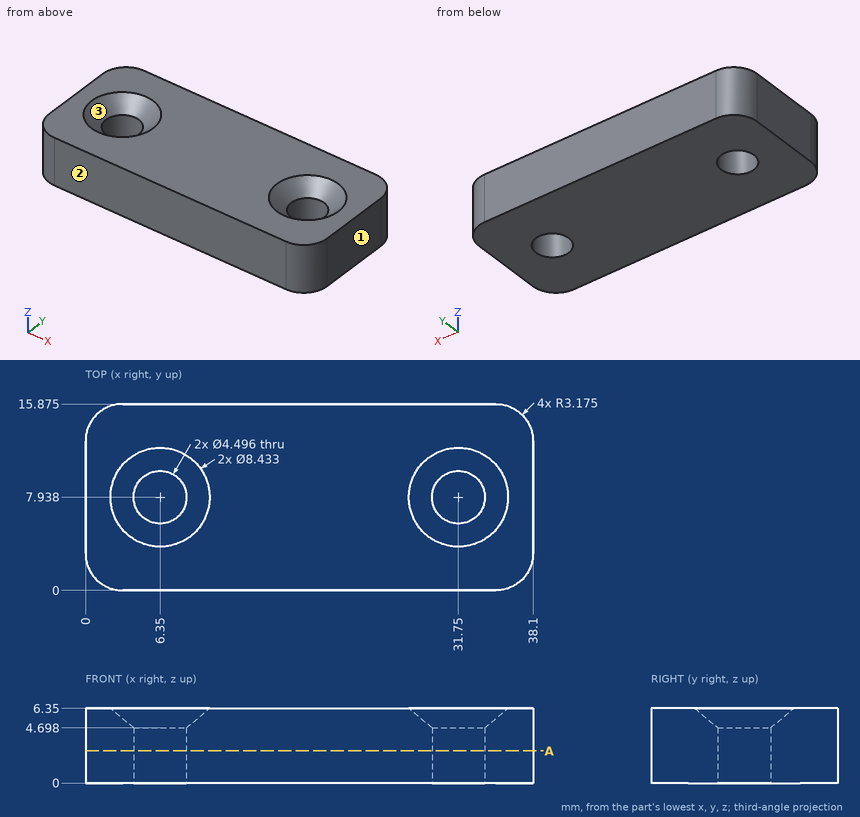
Design review of the part shown in the three views and the two pictorial views. Dimensions are in mm from the part's minimum x, y and z. Round coordinates to 2 decimals unless told otherwise and drop trailing zeros. Use one line per item in the form item = value.
1) Mouldability with a two-part tool opening along Y and no side actions: class the marked faces 1, 2 and 3 as pulls with the +Y half, pulls with the -Y half, needs draft (parallel to the pull), parting line crosses it, or undercut.
Solutions:
face_1 = needs draft
face_2 = pulls with the -Y half
face_3 = undercut
2) Clearance check with a flat-ended pin moving along its axis: P1, Ø1.5, axis at x = 13, z = 1, coming from the -Y side. State where the tip first meets the part, or that it passes through.
Solutions:
P1 = 0
3) We need section A-A on z = 2.75. State how many separate pieces and enclosed holes the cut face has.
Solutions:
separate_pieces = 1
enclosed_holes = 2
4) Wall thickness on probe 1 along Y at (x, z) = (31.75, 2.5) (1 decimal); probe 2 along X at (y, z) = (9, 3.5); probe 3 along X at (y, z) = (3, 3) (1 decimal): over which ranges is each line inside the solid? List them lowest first.
Solutions:
probe_1 = 0 to 5.7, 10.2 to 15.9
probe_2 = 0 to 4.37, 8.33 to 29.77, 33.73 to 38.1
probe_3 = 0 to 38.1
